Verification items for the finished model (mm, model axes). Coordinates: 2 decimals unless noted, no trailing zeros. Write each loop counter-clockwise with the first axis right and the second up, starting at its lowest first coordinate (ties: lowest second). Pieces come first, ordered by that corner, then holes. Notation, with made-up numbers: (22, 48.25) -> (39, 48.25) arc R34 ccw to (39, 87.25) -> close; hole circle Ø2 at (42, 2). An arc over 180 degrees is marked (long way). Use a Markdown table: item, result. Add a question column.
from build123d import *

# Parameters (mm, degrees)
SKETCH1_R               = 4.75
BOSS_EXTRUDE1_DEPTH     = 3.2
SKETCH2_OUTSIDE_W       = 42.576
SKETCH2_OUTSIDE_H       = 45.336
SKETCH2_OUTSIDE_R       = 10.39980339
CUT_EXTRUDE1_DEPTH      = 6.4
CUT_EXTRUDE1_DRAFT      = -45
MIRROR1_COPY_1_SKETCH_W = 42.576
MIRROR1_COPY_1_SKETCH_H = 45.336
MIRROR1_COPY_1_SKETCH_R = 10.39980339
MIRROR1_COPY_1_DEPTH    = 6.4
MIRROR1_COPY_1_DRAFT    = -45


with BuildPart() as part:
    # Sketch1 → Boss-Extrude1 (new, symmetric)
    with BuildSketch(Plane.XY):
        Polygon((10.620274545, -5.605144899), (10.164335146, 6.394855101), (-0.455939398, 12), (-10.620274545, 5.605144899), (-10.164335146, -6.394855101), (0.455939398, -12), align=None)
        Circle(SKETCH1_R, mode=Mode.SUBTRACT)
    extrude(amount=BOSS_EXTRUDE1_DEPTH, both=True)


with BuildPart() as cut_extrude1_tool:
    # Sketch2 outside → Cut-Extrude1 (with draft: the straight prism first)
    with BuildSketch(Plane.XY.offset(3.2)):
        Rectangle(SKETCH2_OUTSIDE_W, SKETCH2_OUTSIDE_H)
        Circle(SKETCH2_OUTSIDE_R, mode=Mode.SUBTRACT)
    extrude(amount=-CUT_EXTRUDE1_DEPTH)
    # Cut-Extrude1: the draft: its side faces are tilted about the plane it starts from
    cut_extrude1_sides = [cut_extrude1_tool.faces().sort_by_distance(p)[0] for p in [
        (0, -22.668, 0),
        (21.288, 0, 0),
        (0, 22.668, 0),
        (-21.288, 0, 0),
        (-10.39980339, 0, 0),
    ]]
    draft(cut_extrude1_sides, Plane.XY.offset(3.2), CUT_EXTRUDE1_DRAFT)


with BuildPart() as part_1:
    add(part.part)

    # Cut-Extrude1: cut by cut_extrude1_tool
    add(cut_extrude1_tool.part, mode=Mode.SUBTRACT)


with BuildPart() as mirror1_copy_1_tool:
    # Mirror1 copy 1 sketch → Mirror1 copy 1 (with draft: the straight prism first)
    with BuildSketch(Plane(origin=(0, 0, -3.2), x_dir=(1, 0, 0), z_dir=(0, 0, -1))):
        Rectangle(MIRROR1_COPY_1_SKETCH_W, MIRROR1_COPY_1_SKETCH_H)
        Circle(MIRROR1_COPY_1_SKETCH_R, mode=Mode.SUBTRACT)
    extrude(amount=-MIRROR1_COPY_1_DEPTH)
    # Mirror1 copy 1: the draft: its side faces are tilted about the plane it starts from
    mirror1_copy_1_sides = [mirror1_copy_1_tool.faces().sort_by_distance(p)[0] for p in [
        (0, -22.668, 0),
        (21.288, 0, 0),
        (0, 22.668, 0),
        (-21.288, 0, 0),
        (-10.39980339, 0, 0),
    ]]
    draft(mirror1_copy_1_sides, Plane(origin=(0, 0, -3.2), x_dir=(1, 0, 0), z_dir=(0, 0, -1)), MIRROR1_COPY_1_DRAFT)


with BuildPart() as part_2:
    add(part_1.part)

    # Mirror1 copy 1: cut by mirror1_copy_1_tool
    add(mirror1_copy_1_tool.part, mode=Mode.SUBTRACT)


solid = part_2.part
1) Gauge pin test, flat ends, axial feed: pin 1 (8.5 mm diameter, centred on x = 0, y = 0, fed in from +Z); pin 2 (6 mm diameter, centred on x = -1.5, y = -1.5, fed in from -Z). Record the tip position at first contact, or that the pin passes through.
2) Release check for a two-part mould opening along Y. For faces 1 (the face through (-9.11, -5.76, -2.82)), 2 (the face through (10.395, 0.311, 0.045)), 3 (the face through (4.5, -2.2, 3.2)), 4 (the face through (2.192, -4.214, -0.045)) record: released by +Y, released by -Y, zero draft, split by the parting line, or undercut.
3) Cross-section at A-A on z = -0.5. Record the boundary of the cut face in (x, y), then the cut area to 3 significant figures.
4) Cross-section at B-B on x = 0. Record the boundary of the cut face in (y, z), then the cut area to 3 significant figures.
5) Cross-section at D-D on z = -2.5. Record the boundary of the cut face in (x, y).
6) Thickness scan on L1, parallel to Y at x = -0.75, z = 0.25 (3 decimals); L2, parallel to Y at x = 0, z = -1.5; L3, parallel to X at y = 4.25, z = -3. Record the ranges inside material, lowest first.
Returned:
| question | item | result |
|---|---|---|
| 1 | pin 1 | passes through |
| 1 | pin 2 | stops at z = -3.2 |
| 2 | face 1 | released by -Y |
| 2 | face 2 | released by +Y |
| 2 | face 3 | zero draft |
| 2 | face 4 | undercut |
| 3 | outline | (-10.62, 5.61) -> (-10.16, -6.39) -> (0.46, -12) -> (10.62, -5.61) -> (10.16, 6.39) -> (-0.46, 12) -> close; hole circle Ø9.5 at (0, 0) |
| 3 | area | 304 mm² |
| 4 | outline | (-11.76, -1.84) -> (-10.4, -3.2) -> (-4.75, -3.2) -> (-4.75, 3.2) -> (-10.4, 3.2) -> (-11.76, 1.84) -> close; (4.75, -3.2) -> (10.4, -3.2) -> (11.76, -1.84) -> (11.76, 1.84) -> (10.4, 3.2) -> (4.75, 3.2) -> close |
| 4 | area | 86.0 mm² |
| 5 | outline | (-10.54, 3.48) -> (-10.25, -4.27) arc R11.1 ccw to (-8.29, -7.39) -> (-1.42, -11.01) arc R11.1 ccw to (2.25, -10.87) -> (8.82, -6.74) arc R11.1 ccw to (10.54, -3.48) -> (10.25, 4.27) arc R11.1 ccw to (8.29, 7.39) -> (1.42, 11.01) arc R11.1 ccw to (-2.25, 10.87) -> (-8.82, 6.74) arc R11.1 ccw to start; hole circle Ø9.5 at (0, 0) |
| 6 | L1 | y = -11.364 to -4.69, 4.69 to 11.815 |
| 6 | L2 | y = -11.76 to -4.75, 4.75 to 11.76 |
| 6 | L3 | x = -9.71 to -2.12, 2.12 to 9.71 |
